```python
from build123d import *

# Parameters (mm, degrees)
SKETCH1_W           = 120
SKETCH1_H           = 60
BOSS_EXTRUDE1_DEPTH = 5
SKETCH2_R           = 11.375
CUT_EXTRUDE1_DEPTH  = 68.268120235
FILLET1_R           = 5
SKETCH3_R           = 1.5
CUT_EXTRUDE2_DEPTH  = 68.268120235
SKETCH4_R           = 2.875
CUT_EXTRUDE3_DEPTH  = 2.5
CHAMFER1_SIZE       = 1
SKETCH5_R           = 16
CUT_EXTRUDE4_DEPTH  = 3
SKETCH6_R           = 2.5
BOSS_EXTRUDE2_DEPTH = 0.15


with BuildPart() as part:
    # Sketch1 → Boss-Extrude1 (new body)
    with BuildSketch(Plane.XY):
        Rectangle(SKETCH1_W, SKETCH1_H)
    extrude(amount=BOSS_EXTRUDE1_DEPTH)

    # Sketch2 → Cut-Extrude1 (cut, through all)
    with BuildSketch(Plane.XY.offset(5)):
        Circle(SKETCH2_R)
        with Locations((37.5, 0)):
            Circle(SKETCH2_R)
        with Locations((-37.5, 0)):
            Circle(SKETCH2_R)
    extrude(amount=-CUT_EXTRUDE1_DEPTH, mode=Mode.SUBTRACT)

    # Fillet1
    fillet1_edges = [part.edges().sort_by_distance(p)[0] for p in [
        (60, -30, 2.5),
        (-60, -30, 2.5),
        (-60, 30, 2.5),
        (60, 30, 2.5),
    ]]
    fillet(fillet1_edges, radius=FILLET1_R)

    # Sketch3 → Cut-Extrude2 (cut, through all)
    with BuildSketch(Plane.XY.offset(5)):
        with Locations((-55, 25)):
            Circle(SKETCH3_R)
        with Locations((55, 25)):
            Circle(SKETCH3_R)
        with Locations((55, -25)):
            Circle(SKETCH3_R)
        with Locations((-55, -25)):
            Circle(SKETCH3_R)
    extrude(amount=-CUT_EXTRUDE2_DEPTH, mode=Mode.SUBTRACT)

    # Sketch4 → Cut-Extrude3 (cut)
    with BuildSketch(Plane.XY.offset(5)):
        with Locations((-55, 25)):
            Circle(SKETCH4_R)
        with Locations((55, 25)):
            Circle(SKETCH4_R)
        with Locations((55, -25)):
            Circle(SKETCH4_R)
        with Locations((-55, -25)):
            Circle(SKETCH4_R)
    extrude(amount=-CUT_EXTRUDE3_DEPTH, mode=Mode.SUBTRACT)

    # Chamfer1
    chamfer1_edges = [part.edges().sort_by_distance(p)[0] for p in [
        (0, -30, 5),
        (-60, 0, 5),
        (60, 0, 5),
        (0, 30, 5),
        (-58.535533906, 28.535533906, 5),
        (58.535533906, 28.535533906, 5),
        (58.535533906, -28.535533906, 5),
        (-58.535533906, -28.535533906, 5),
    ]]
    chamfer(chamfer1_edges, length=CHAMFER1_SIZE)

    # Sketch5 → Cut-Extrude4 (cut)
    with BuildSketch(Plane(origin=(0, 0, 0), x_dir=(-1, 0, 0), z_dir=(0, 0, -1))):
        with Locations((-37.5, 0)):
            Circle(SKETCH5_R)
        Circle(SKETCH5_R)
        with Locations((37.5, 0)):
            Circle(SKETCH5_R)
    extrude(amount=-CUT_EXTRUDE4_DEPTH, mode=Mode.SUBTRACT)

    # Sketch6 → Boss-Extrude2 (add)
    with BuildSketch(Plane.XY.offset(2.5)):
        with Locations((-55, 25)):
            Circle(SKETCH6_R)
        with Locations((55, 25)):
            Circle(SKETCH6_R)
        with Locations((55, -25)):
            Circle(SKETCH6_R)
        with Locations((-55, -25)):
            Circle(SKETCH6_R)
    extrude(amount=-BOSS_EXTRUDE2_DEPTH)


solid = part.part
```
Input: part model. Units: mm. Frame: model coordinates. A direction names the side the tool comes from. Give positions to 0.01 mm unless a question says otherwise; leave off trailing zeros. Loops run counter-clockwise (first coordinate to the right, second up) from the corner with the lowest first, then second, coordinate; pieces in that order, holes last. Notation, with made-up numbers: M 77.25,-3.5 L 134.25,-3.5 A19 cw 134.25,14.5 Z; hole C -13.5,-7.75 d7. An arc over 180 degrees is marked long. Answer as CSV lines item,"result". Start each with the question number.
1. Pull-direction query (Y, two-part tool) for faces 4 (the face through (12, 0, 5)), 5 (the face through (58, 29, 2)), 6 (the face through (-57.28, -26.75, 3.77)); classes: released by +Y, released by -Y, zero draft, split by the parting line, or undercut.
2. Pin query (flat end, axial travel): P1, Ø16, axis at x = 31, y = -5.5, coming from the -Z side; P2, Ø2.5, axis at x = -55, y = -25, coming from the -Z side; P3, Ø3, axis at x = -56, y = -25, coming from the +Z side. Return the tip coordinate at first contact, or that it passes through.
3. Section A-A on y = 0. State how many separate pieces and enclosed holes the cut face has, plus the area to 4 significant figures.
4. Reachability of faces 1 (the face through (-57.28, 23.25, 3.77)), 2 (the face through (-58.063, -27.996, 4.715)), 3 (the face through (4, 11, 3)) from +Z, -Z, +X, -X, +Y, -Y: full face, straight path, thin tool, end or side. Return the list, or none.
5. Section D-D on y = -14. Return loops of the section in (x, z), plus the area to 3 significant figures.
6. Line query: L1, parallel to X at y = -6.5, z = 3.55; L2, parallel to X at y = 11, z = 2.75; L3, parallel to Y at x = 37.5, z = 1.15. Output: solid intervals per line, ascending.
7. Section C-C on z = 1.2. Return loops of the section in (x, y).
8. Section B-B on x = 37.5. Return loops of the section in (y, z) (3 decimals), plus the area to 4 significant figures.
Computed values:
1,face 4,"zero draft"
1,face 5,"released by +Y"
1,face 6,"undercut"
2,P1,"stops at z = 0"
2,P2,"stops at z = 2.35"
2,P3,"stops at z = 2.5"
3,separate pieces,"4"
3,enclosed holes,"0"
3,area,"174.5 mm²"
4,face 1,"+Z"
4,face 2,"+Z, -X, -Y"
4,face 3,"-Z"
5,outline,"M -60,0 L -45.25,0 L -45.25,3 L -29.75,3 L -29.75,0 L -7.75,0 L -7.75,3 L 7.75,3 L 7.75,0 L 29.75,0 L 29.75,3 L 45.25,3 L 45.25,0 L 60,0 L 60,4 L 59,5 L -59,5 L -60,4 Z"
5,area,"460 mm²"
6,L1,"x = -60 to -46.83, -28.17 to -9.33, 9.33 to 28.17, 46.83 to 60"
6,L2,"x = -60 to -49.12, -25.88 to -11.62, 11.62 to 25.88, 49.12 to 60"
6,L3,"y = -30 to -16, 16 to 30"
7,outline,"M -60,-25 A5 ccw -55,-30 L 55,-30 A5 ccw 60,-25 L 60,25 A5 ccw 55,30 L -55,30 A5 ccw -60,25 Z; hole C -55,-25 d3; hole C -55,25 d3; hole C -37.5,0 d32; hole C 0,0 d32; hole C 37.5,0 d32; hole C 55,-25 d3; hole C 55,25 d3"
8,outline,"M -30,0 L -16,0 L -16,3 L -11.375,3 L -11.375,5 L -29,5 L -30,4 Z; M 11.375,3 L 16,3 L 16,0 L 30,0 L 30,4 L 29,5 L 11.375,5 Z"
8,area,"157.5 mm²"
